from build123d import *

# Parameters (mm, degrees)
F0_R     = 12.5
F1_DEPTH = 10


with BuildPart() as f1:
    # F0 (on Top) → F1 (new body)
    with BuildSketch(Plane.XY):
        with BuildLine():
            ThreePointArc((0, 17.5), (5.125631, 5.125631), (17.5, 0))
            Line((17.5, 0), (57, 0))
            ThreePointArc((57, 0), (60.535534, 1.464466), (62, 5))
            Line((62, 5), (62, 30))
            ThreePointArc((62, 30), (60.535534, 33.535534), (57, 35))
            Line((57, 35), (17.5, 35))
            ThreePointArc((17.5, 35), (5.125631, 29.874369), (0, 17.5))
        make_face()
        with Locations((17.5, 17.5)):
            Circle(F0_R, mode=Mode.SUBTRACT)
    extrude(amount=F1_DEPTH)

    # F2 (on face) → F3 (revolve, cut)
    with BuildSketch(Plane.XY.offset(10)):
        with BuildLine():
            Line((37, 24.5), (37, 8))
            Line((37, 8), (40, 8))
            Line((40, 8), (40, 24.5))
            Line((40, 24.5), (42, 24.5))
            Line((42, 24.5), (42, 25.25))
            ThreePointArc((42, 25.25), (41.12132, 27.37132), (39, 28.25))
            Line((39, 28.25), (37, 28.25))
            Line((37, 28.25), (37, 24.5))
        make_face()
    revolve(axis=Axis((37, 16.25, 10), (0, 1, 0)), mode=Mode.SUBTRACT)

    # F2 (on face) → F4 (revolve, cut)
    with BuildSketch(Plane.XY.offset(10)):
        with BuildLine():
            Line((52, 24.5), (52, 8))
            Line((52, 8), (55, 8))
            Line((55, 8), (55, 24.5))
            Line((55, 24.5), (57, 24.5))
            Line((57, 24.5), (57, 25.25))
            ThreePointArc((57, 25.25), (56.12132, 27.37132), (54, 28.25))
            Line((54, 28.25), (52, 28.25))
            Line((52, 28.25), (52, 24.5))
        make_face()
    revolve(axis=Axis((52, 16.25, 10), (0, 1, 0)), mode=Mode.SUBTRACT)


solid = f1.part
The listing builds one solid part. Answer for the finished solid, in the listing's coordinates (mm). A direction names the side the tool comes from. Give positions to 0.01 mm unless a question says otherwise; leave off trailing zeros. Write each loop counter-clockwise with the first axis right and the second up, starting at its lowest first coordinate (ties: lowest second). Pieces come first, ordered by that corner, then holes.
Item 1: Section B-B, the plane x = 10 is taken. Write down the section's boundary in (y, z).
Item 2: Which of the six approach directions +Z, -Z, +X, -X, +Y, -Y give full straight-line access (tool end or side, diameter ignored) to faces 1 (the cylindrical face through (14.79, 5.297, 4.93)), 2 (the flat face through (37, 8, 9))?
Item 3: Determine the mould class of faces 3 (the flat face through (37, 0, 5)), 4 (the flat face through (37, 28.25, 9)), 5 (the flat face through (31, 18, 10)) for opening direction Y: released by +Y, released by -Y, zero draft, split by the parting line, or undercut.
Item 4: Find the intervals of material crossed by line 1 along Y through (x, z) = (17.5, 4.25); line 2 along X through (y, z) = (9.5, 9.75); line 3 along X through (y, z) = (24, 8), in increasing order.
Item 5: Section A-A, the plane z = 1 is taken. Write down the section's boundary in (x, y), plus the area to 3 significant figures.
Item 6: Section C-C, the plane y = 23 is taken. Write down the section's boundary in (x, z).
Item 7: Section D-D, the plane x = 21 is taken. Write down the section's boundary in (y, z), plus the area to 3 significant figures.
Completed:
1. outline: (1.69, 0) - (7.5, 0) - (7.5, 10) - (1.69, 10) - close; (27.5, 0) - (33.31, 0) - (33.31, 10) - (27.5, 10) - close
2. face 1: +Z, -Z
2. face 2: +Z
3. face 3: released by -Y
3. face 4: undercut
3. face 5: zero draft
4. line 1: y = 0 to 5, 30 to 35
4. line 2: x = 1.94 to 7.9, 27.1 to 34.01, 39.99 to 49.01, 54.99 to 62
4. line 3: x = 1.25 to 6.82, 28.18 to 34.76, 39.24 to 49.76, 54.24 to 62
5. outline: (0, 17.5) arc R17.5 ccw to (17.5, 0) - (57, 0) arc R5 ccw to (62, 5) - (62, 30) arc R5 ccw to (57, 35) - (17.5, 35) arc R17.5 ccw to start; hole circle Ø25 at (17.5, 17.5)
5. area: 1,540 mm2
6. outline: (0.89, 0) - (6.28, 0) - (6.28, 10) - (0.89, 10) - close; (28.72, 0) - (62, 0) - (62, 10) - (55, 10) arc R3 cw to (49, 10) - (40, 10) arc R3 cw to (34, 10) - (28.72, 10) - close
7. outline: (0, 0) - (5.5, 0) - (5.5, 10) - (0, 10) - close; (29.5, 0) - (35, 0) - (35, 10) - (29.5, 10) - close
7. area: 110 mm2
